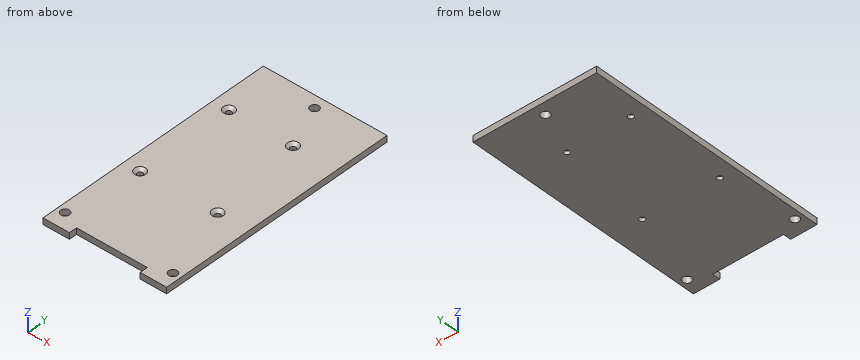
Autodesk Inventor part; units mm, degrees
ref_plane "YZ Plane" through (0, 0, 0) normal (1, 0, 0) x (0, 1, 0)
ref_plane "XZ Plane" through (0, 0, 0) normal (0, 1, 0) x (-1, 0, 0)
ref_plane "XY Plane" through (0, 0, 0) normal (0, 0, 1) x (1, 0, 0)
sketch "Sketch2" plane through (0, 0, 0) normal (0, 0, 1) x (1, 0, 0)
  line L0 (39.25, -77.5) -> (-39.25, -77.5)
  line L1 (-39.25, -77.5) -> (-39.25, 77.5)
  line L2 (-39.25, 77.5) -> (39.25, 77.5)
  line L3 (39.25, 77.5) -> (39.25, -77.5)
  line L4 (39.25, -77.5) -> (-39.25, 77.5) construction
  line L5 (-39.25, -77.5) -> (39.25, 77.5) construction
  point P0 (0, 0)
  dimension "d0" = 78.5
  dimension "d1" = 155
extrude "Extrusion1" add sketch "Sketch2" along normal blind 4
sketch "Sketch3" plane through (0, 0, 4) normal (0, 0, 1) x (1, 0, 0)
  line L0 (0, 108.5) -> (0, -108.5) construction
  line L1 (39.25, 77.5) -> (-39.25, 77.5) construction
  point P0 (0, 0)
  point P1 (0, 70)
  point P2 (-34.25, -67.5)
  point P3 (34.25, -67.5)
  dimension "d4" = 34.25
  dimension "d5" = 34.25
  dimension "d6" = 137.5
  dimension "d8" = 7.5
  dimension "d9" = 137.5
hole "Hole1" at (0, 70, 4) at (-34.25, -67.5, 4) at (34.25, -67.5, 4) direction (0, 0, -1) diameter 5.5 depth 9.5
sketch "Sketch4" plane through (0, 0, 0) normal (0, 0, -1) x (-1, 0, 0)
  line L0 (-27.565, 44.5) -> (-27.565, 40.5) construction
  line L1 (-27.565, 40.5) -> (-37.565, 40.5) construction
  line L2 (-37.565, 40.5) -> (-37.565, 32.5) construction
  line L3 (-37.565, 32.5) -> (-27.565, 32.5) construction
  line L4 (-27.565, 32.5) -> (-27.565, -48.52) construction
  line L5 (-27.565, -48.52) -> (-10.565, -48.52) construction
  line L6 (-10.565, -48.52) -> (-10.565, -58.52) construction
  line L7 (-10.565, -58.52) -> (-2.565, -58.52) construction
  line L8 (-2.565, -58.52) -> (-2.565, -48.52) construction
  line L9 (-2.565, -48.52) -> (37.5, -48.52) construction
  line L10 (37.5, -48.52) -> (37.5, 44.5) construction
  line L11 (37.5, 44.5) -> (28.5, 44.5) construction
  line L12 (28.5, 44.5) -> (26.5, 46.5) construction
  line L13 (26.5, 46.5) -> (18.5, 46.5) construction
  line L14 (18.5, 46.5) -> (18.5, 56.5) construction
  line L15 (18.5, 56.5) -> (7.5, 56.5) construction
  line L16 (7.5, 56.5) -> (7.5, 46.5) construction
  line L17 (7.5, 46.5) -> (-6.565, 46.5) construction
  line L18 (-6.565, 46.5) -> (-8.565, 44.5) construction
  line L19 (-8.565, 44.5) -> (-27.565, 44.5) construction
  circle A0 centre (29.081, 42.025) radius 1.6 construction
  circle A1 centre (-11.625, 42.025) radius 1.6 construction
  circle A2 centre (28.95, -20.606) radius 1.6 construction
  circle A3 centre (-19.179, -19.336) radius 1.6 construction
  point P0 (0, 0)
hole "Hole2" at (-29.081, 42.025, 0) at (-28.95, -20.606, 0) at (19.179, -19.336, 0) at (11.625, 42.025, 0) direction (0, 0, 1) diameter 3.5 depth 9.5
chamfer "Chamfer1" distance 1.8 angle 45 4 edges at (-28.95, -22.356, 4) (19.179, -21.086, 4) (-29.081, 40.275, 4) (11.625, 40.275, 4)
sketch "Sketch6" plane through (0, 0, 4) normal (0, 0, 1) x (1, 0, 0)
  circle A0 centre (-28.95, -20.606) radius 3.55 construction
  circle A1 centre (11.625, 42.025) radius 3.55 construction
  circle A2 centre (-34.25, -67.5) radius 2.75 construction
  circle A3 centre (0, 70) radius 2.75 construction
  circle A4 centre (34.25, -67.5) radius 2.75 construction
  line L0 (39.25, 77.5) -> (-39.25, 77.5) construction
  line L1 (-39.25, 77.5) -> (-39.25, -77.5) construction
  line L2 (-39.25, -77.5) -> (39.25, -77.5) construction
  line L3 (39.25, -77.5) -> (39.25, 77.5) construction
  circle A5 centre (19.179, -19.336) radius 3.55 construction
  circle A6 centre (-29.081, 42.025) radius 3.55 construction
  line L4 (22.5, -72.5) -> (-22.5, -72.5)
  line L5 (-22.5, -72.5) -> (-22.5, -77.5)
  line L6 (-22.5, -77.5) -> (22.5, -77.5)
  line L7 (22.5, -77.5) -> (22.5, -72.5)
  line L8 (0, 108.5) -> (0, -108.5) construction
  point P0 (0, 0)
  dimension "d33" = 45
  dimension "d34" = 5
  dimension "d35" = 22.5
extrude "Extrusion3" cut sketch "Sketch6" against normal blind 10
equation "\"d35\" = 0.5 * d33"
properties part number "P042_BoitierCouvercleV4_moduleHaut"
Could you check a few things on this model? Use its own coordinates, in mm. Give positions to 0.01 mm unless a question says otherwise; leave off trailing zeros. Order: outer loops, then holes, each group sorted by start corner. A loop starts at its lowest first (then second) coordinate and runs counter-clockwise, first axis right, second up.
Item 1: I'm going to push flat-ended pins straight in: pin 1 (4 mm diameter, centred on x = -28.95, y = -20.606, fed in from -Z); pin 2 (4 mm diameter, centred on x = 19.179, y = -19.336, fed in from +Z). Where does each tip first touch, or does it pass through?
Item 2: I need wall thicknesses on line 1 (X direction, y = -67.5, z = 2.85); line 2 (X direction, y = 70, z = 2.45); line 3 (Y direction, x = -28.95, z = 1.7). Which ranges of each line are inside material? Lowest first, please.
Item 3: If we section it at B-B, the plane y = 70: Write out the boundary of the cut face in (x, z), plus the area to 3 significant figures.
Item 4: If we section it at C-C, the plane x = -14: Write out the boundary of the cut face in (y, z), plus the area to 3 significant figures.
Item 5: If we section it at A-A, the plane x = 34.25: Write out the boundary of the cut face in (y, z), plus the area to 3 significant figures.
Values:
1. pin 1: stops at z = 0
1. pin 2: stops at z = 2.45
2. line 1: x = -39.25 to -37, -31.5 to 31.5, 37 to 39.25
2. line 2: x = -39.25 to -2.75, 2.75 to 39.25
2. line 3: y = -77.5 to -22.36, -18.86 to 40.28, 43.77 to 77.5
3. outline: (-39.25, 0) - (-2.75, 0) - (-2.75, 4) - (-39.25, 4) - close; (2.75, 0) - (39.25, 0) - (39.25, 4) - (2.75, 4) - close
3. area: 292 mm2
4. outline: (-72.5, 0) - (77.5, 0) - (77.5, 4) - (-72.5, 4) - close
4. area: 600 mm2
5. outline: (-77.5, 0) - (-70.25, 0) - (-70.25, 4) - (-77.5, 4) - close; (-64.75, 0) - (77.5, 0) - (77.5, 4) - (-64.75, 4) - close
5. area: 598 mm2
